from build123d import *

# Parameters (mm, degrees)
SKETCH_1_W             = 120
SKETCH_1_H             = 120
EXTRUDE_1_DEPTH        = 5
SKETCH_2_W             = 60
SKETCH_2_H             = 60
SKETCH_2_W_2           = 54
SKETCH_2_H_2           = 54
EXTRUDE_2_DEPTH        = 2000
FILLET_1_R             = 5
SKETCH_3_R             = 5
CUT_EXTRUDE_1_DEPTH    = 2000
EXTRUDE_5_DEPTH        = 7.5
PATTERN_LINEAR_1_COUNT = 2
PATTERN_LINEAR_1_PITCH = 1500
SKETCH_7_R             = 12.5
EXTRUDE_6_DEPTH        = 30
SKETCH_8_R             = 4
EXTRUDE_7_DEPTH        = 35
PATTERN_LINEAR_2_COUNT = 2
PATTERN_LINEAR_2_PITCH = 1500


with BuildPart() as part:
    # Sketch 1 → Extrude 1 (new body)
    with BuildSketch(Plane(origin=(0, 0, 0), x_dir=(1, 0, 0), z_dir=(0, 1, 0))):
        Rectangle(SKETCH_1_W, SKETCH_1_H)
    extrude(amount=EXTRUDE_1_DEPTH)

    # Sketch 2 → Extrude 2 (add)
    with BuildSketch(Plane(origin=(0, 5, 0), x_dir=(1, 0, 0), z_dir=(0, 1, 0))):
        Rectangle(SKETCH_2_W, SKETCH_2_H)
        Rectangle(SKETCH_2_W_2, SKETCH_2_H_2, mode=Mode.SUBTRACT)
    extrude(amount=EXTRUDE_2_DEPTH)

    # Fillet 1
    fillet_1_edges = [part.edges().sort_by_distance(p)[0] for p in [
        (30, 1005, -30),
        (-30, 1005, -30),
        (-30, 1005, 30),
        (30, 1005, 30),
    ]]
    fillet(fillet_1_edges, radius=FILLET_1_R)

    # Sketch 3 → Cut-Extrude 1 (cut)
    with BuildSketch(Plane(origin=(0, 5, 0), x_dir=(1, 0, 0), z_dir=(0, 1, 0))):
        with Locations(Location((-45, 45, 0), (0, 0, 270))):
            Circle(SKETCH_3_R)
        with Locations(Location((45, 45, 0), (0, 0, 270))):
            Circle(SKETCH_3_R)
        with Locations(Location((-45, -45, 0), (0, 0, 270))):
            Circle(SKETCH_3_R)
        with Locations(Location((45, -45, 0), (0, 0, 270))):
            Circle(SKETCH_3_R)
    extrude(amount=-CUT_EXTRUDE_1_DEPTH, mode=Mode.SUBTRACT)

    # Sketch 6 → Extrude 5 (add, symmetric)
    with BuildSketch(Plane(origin=(0, 0, 0), x_dir=(0, 0, -1), z_dir=(1, 0, 0))):
        Polygon((30, 1785), (30, 1725), (40, 1725), (40, 1755), (33, 1755), (33, 1785), align=None)
    extrude_5 = extrude(amount=EXTRUDE_5_DEPTH, both=True)

    # Pattern Linear 1: Extrude 5 ×2
    with Locations(*[(0, -i * PATTERN_LINEAR_1_PITCH, 0) for i in range(1, PATTERN_LINEAR_1_COUNT)]):
        add(extrude_5)

    # Sketch 7 → Extrude 6 (add)
    with BuildSketch(Plane(origin=(0, 1755, 0), x_dir=(1, 0, 0), z_dir=(0, 1, 0))):
        with Locations((0, 52)):
            Circle(SKETCH_7_R)
    extrude_6 = extrude(amount=-EXTRUDE_6_DEPTH)

    # Sketch 8 → Extrude 7 (add)
    with BuildSketch(Plane(origin=(0, 1755, 0), x_dir=(1, 0, 0), z_dir=(0, 1, 0))):
        with Locations(Location((0, 50, 0), (0, 0, 90))):
            Circle(SKETCH_8_R)
    extrude_7 = extrude(amount=EXTRUDE_7_DEPTH)

    # Pattern Linear 2: Extrude 6, Extrude 7 ×2
    with Locations(*[(0, -i * PATTERN_LINEAR_2_PITCH, 0) for i in range(1, PATTERN_LINEAR_2_COUNT)]):
        add(extrude_6)
        add(extrude_7)


solid = part.part
Check sheet for the modelled part. Datum: model origin and axes. Units: mm. A direction names the side the tool comes from. Give positions to 0.01 mm unless a question says otherwise; leave off trailing zeros. Order: outer loops, then holes, each group sorted by start corner. A loop starts at its lowest first (then second) coordinate and runs counter-clockwise, first axis right, second up. Notation, with made-up numbers: M 2,57 L 57,57 A27 cw 57,94 Z; hole C 75.25,62.25 d11. An arc over 180 degrees is marked long. Answer as CSV lines item,"result". Start each with the question number.
Item 1: Thickness scan on line 1 (X direction, y = 1, z = -45); line 2 (Y direction, x = 3.5, z = -51); line 3 (Z direction, x = 4.5, y = 811.5). Record the ranges inside material, lowest first. Write a range as [from, to].
Item 2: Mould release check, pull along Z, two halves, no side actions. Record for faces 1 (the face through (0, 991, 30)), 2 (the face through (0, 991, 27)), 3 (the face through (-30, 991, 0)): +Z half, -Z half, draft (parallel to the pull), parting line (faces both ways), or undercut.
Item 3: Cross-section at A-A on y = 772. Enter the section's corners in (x, z).
Item 4: Gauge pin test, flat ends, axial feed: P1, Ø4, axis at x = -0.5, z = -51.5, coming from the +Y side; P2, Ø6, axis at y = 1271, z = -32, coming from the -X side; P3, Ø6, axis at x = -30, y = 328, coming from the -Z side. Record the tip position at first contact, or that the pin passes through.
Item 5: Cross-section at B-B on z = 2. Enter the section's corners in (x, y).
Item 6: Tool access check on faces 4 (the face through (30, 991, 0)), 5 (the face through (-27, 991, 0)), 6 (the face through (0, 2005, -29)). Record the directions out of +Z, -Z, +X, -X, +Y, -Y that give a thin tool (end or side, any length) a straight path to the whole face; none if there is none.
Established:
1,line 1,"x = [-60, -50], [-40, 40], [50, 60]"
1,line 2,"y = [0, 5], [225, 290], [1725, 1790]"
1,line 3,"z = [-30, -27], [27, 30]"
2,face 1,"+Z half"
2,face 2,"undercut"
2,face 3,"draft"
3,outline,"M -30,-25 A5 ccw -25,-30 L 25,-30 A5 ccw 30,-25 L 30,25 A5 ccw 25,30 L -25,30 A5 ccw -30,25 Z; hole M -27,-27 L 27,-27 L 27,27 L -27,27 Z"
4,P1,"stops at y = 1790"
4,P2,"stops at x = -28"
4,P3,"stops at z = -29.58"
5,outline,"M -60,0 L 60,0 L 60,5 L 30,5 L 30,2005 L 27,2005 L 27,5 L -27,5 L -27,2005 L -30,2005 L -30,5 L -60,5 Z"
6,face 4,"+Z, -Z, +X, +Y"
6,face 5,"+Y"
6,face 6,"+Z, -Z, +X, -X, +Y"
